Autodesk Inventor part; units mm, degrees
ref_plane "YZ Plane" through (0, 0, 0) normal (1, 0, 0) x (0, 1, 0)
ref_plane "XZ Plane" through (0, 0, 0) normal (0, 1, 0) x (-1, 0, 0)
ref_plane "XY Plane" through (0, 0, 0) normal (0, 0, 1) x (1, 0, 0)
sketch "Sketch1" plane through (0, 0, 0) normal (0, 0, 1) x (1, 0, 0)
  circle A0 centre (0, 0) radius 15.9766
  line L0 (0, 0) -> (36.9062, 0)
  circle A1 centre (36.9062, 0) radius 15.9766
  line L1 (36.9062, 0) -> (49.6062, 0)
  line L2 (36.9062, 0) -> (36.9062, 15.9766)
  line L3 (36.9062, 0) -> (36.9062, -15.9766)
  arc A2 (36.9062, -15.9766) -> (36.9062, 15.9766) centre (33.2069, 0) ccw
  circle A3 centre (36.9062, 0) radius 5.08
  circle A4 centre (0, 0) radius 5.08
  line L4 (0, 15.9766) -> (36.9062, 15.9766)
  line L5 (36.9062, -15.9766) -> (0, -15.9766)
  line L6 (31.8262, 0) -> (31.8262, 5.08)
  line L7 (31.8262, 5.08) -> (35.0012, 5.08)
  line L8 (35.0012, 5.08) -> (38.8112, 5.08)
  line L9 (38.8112, 5.08) -> (38.8112, -2.54)
  line L10 (38.8112, -2.54) -> (35.0012, -2.54)
  line L11 (35.0012, -2.54) -> (35.0012, 5.08)
  line L12 (36.9062, 5.08) -> (31.8262, 8.89)
  circle A5 centre (31.8262, 8.89) radius 2.54
  point P0 (35.0012, 4.7093)
  point P1 (38.8112, 4.7093)
  dimension "d3" = 10.16
  dimension "d0" = 31.9532
  dimension "d1" = 36.9062
  dimension "d2" = 12.7
  dimension "d4" = 10.16
  dimension "d5" = 3.175
  dimension "d6" = 3.81
  dimension "d7" = 7.62
  dimension "d12" = 6.35
  dimension "d13" = 5.08
extrude "Extrusion1" add sketch "Sketch1" along normal blind 1.5875 contours A0 | L0 A1 L5 A0 | A0 L4 A1 L0 | A1 L2 L8 L7 L6 L0 | L0 A3 L3 A1 | A2 L1 A3 L9 L8 L2 | L3 A3 L1 A2 | L6 L7 L11 A3 | A3 L9 L1 L2 | L8 L9 A3 | L2 L0 L11 A3 | A3 L11 L8 | L0 L3 L10 L11 | L1 L9 L10 L3
fillet "Fillet1" radius 1.5875 2 edges at (38.8112, -2.54, 0.7937) (35.0012, -2.54, 0.7937)
fillet "Fillet2" radius 0.7937 2 edges at (35.0012, 4.7093, 0.7937) (38.8112, 4.7093, 0.7937)
properties part number "new_winch_pto_poly"
The model under review builds one solid part; all positions refer to its coordinate system, in mm. A direction names the side the tool comes from. Give positions to 0.01 mm unless a question says otherwise; leave off trailing zeros. Loops run counter-clockwise (first coordinate to the right, second up) from the corner with the lowest first, then second, coordinate; pieces in that order, holes last. Notation, with made-up numbers: (-31, 89) -> (5, 89) arc R27 ccw to (5, 128) -> close; hole circle Ø2 at (60, -40). An arc over 180 degrees is marked (long way). Put each result on its own line as item: value. Start each with the question number.
1. We need section B-B on y = 1. State the section outline as (x, z) points, then the cut area to 3 significant figures.
2. Clearance check with a flat-ended pin moving along its axis: P1, Ø0.5, axis at y = 1, z = 0.5, coming from the +X side. State where the tip first meets the part, or that it passes through.
3. We need section D-D on y = 13. State the section outline as (x, z) points.
4. We need section C-C on y = 8.89. State the section outline as (x, z) points, then the cut area to 3 significant figures.
5. We need section A-A on z = 1.3. State the section outline as (x, y) points (1 decimal), then the cut area to 3 significant figures.
6. Wall thickness on probe 1 along Y at (x, z) = (0, 1.15); probe 2 along X at (y, z) = (1, 0.2); probe 3 along X at (y, z) = (8.89, 1.3): over which ranges is each line inside the solid? List them lowest first.
7. For faces 1 (the face through (34.56, 4.04, 0.8)), 2 (the face through (49.603, 0.308, 0.783)), list the 3-axis set-ups (+Z, -Z, +X, -X, +Y, -Y) from which the entire face can be reached by the end or side of a thin tool; tool diameter is ignored.
8. Mouldability with a two-part tool opening along Y and no side actions: class faces 3 (the face through (39.27, 4.05, 0.8)), 4 (the face through (19, -15.977, 1)), 5 (the face through (18, 15.977, 1)) as released by +Y, released by -Y, zero draft, split by the parting line, or undercut.
Determined:
1. outline: (-15.95, 0) -> (-4.98, 0) -> (-4.98, 1.59) -> (-15.95, 1.59) -> close; (4.98, 0) -> (31.93, 0) -> (31.93, 1.59) -> (4.98, 1.59) -> close; (35, 0) -> (38.81, 0) -> (38.81, 1.59) -> (35, 1.59) -> close; (41.89, 0) -> (49.58, 0) -> (49.58, 1.59) -> (41.89, 1.59) -> close
1. area: 78.4 mm^2
2. P1: x = 49.59
3. outline: (-9.29, 0) -> (43.2, 0) -> (43.2, 1.59) -> (-9.29, 1.59) -> close
4. outline: (-13.27, 0) -> (29.29, 0) -> (29.29, 1.59) -> (-13.27, 1.59) -> close; (34.37, 0) -> (46.99, 0) -> (46.99, 1.59) -> (34.37, 1.59) -> close
4. area: 87.6 mm^2
5. outline: (0, -16) -> (36.9, -16) arc R16.4 ccw to (36.9, 16) -> (0, 16) arc R16 ccw to start; hole circle Ø10.2 at (0, 0); hole circle Ø5.1 at (31.8, 8.9); hole (33.7, 3.9) arc R5.1 ccw (long way) to (40.1, 3.9) arc R0.8 ccw to (38.8, 3.3) -> (38.8, -1) arc R1.6 cw to (37.2, -2.5) -> (36.6, -2.5) arc R1.6 cw to (35, -1) -> (35, 3.3) arc R0.8 ccw to start
5. area: 1,730 mm^2
6. probe 1: -15.98 to -5.08, 5.08 to 15.98
6. probe 2: -15.95 to -4.98, 4.98 to 31.93, 35 to 38.81, 41.89 to 49.58
6. probe 3: -13.27 to 29.29, 34.37 to 46.99
7. face 1: +Z, -Z
7. face 2: +Z, -Z, +X
8. face 3: undercut
8. face 4: released by -Y
8. face 5: released by +Y
